```python
from build123d import *

# Parameters (mm, degrees)
CROQUIS1_W              = 34
CROQUIS1_H              = 34
CROQUIS1_R              = 1
SALIENTE_EXTRUIR1_DEPTH = 1
CROQUIS2_W              = 9.310717014
CROQUIS2_H              = 8.671746239
CROQUIS2_W_2            = 1.095378472
CROQUIS2_H_2            = 1.688708478
CROQUIS2_W_3            = 1.004096933
CROQUIS2_H_3            = 1.734349248
SALIENTE_EXTRUIR2_DEPTH = 1


with BuildPart() as part:
    # Croquis1 → Saliente-Extruir1 (new body)
    with BuildSketch(Plane.XY):
        with Locations((17, 17)):
            Rectangle(CROQUIS1_W, CROQUIS1_H)
        with Locations((1.5, 32.5)):
            Circle(CROQUIS1_R, mode=Mode.SUBTRACT)
        with Locations((32.5, 32.5)):
            Circle(CROQUIS1_R, mode=Mode.SUBTRACT)
        with Locations((1.5, 1.5)):
            Circle(CROQUIS1_R, mode=Mode.SUBTRACT)
        with Locations((32.5, 1.5)):
            Circle(CROQUIS1_R, mode=Mode.SUBTRACT)
    extrude(amount=SALIENTE_EXTRUIR1_DEPTH)

    # Croquis2 → Saliente-Extruir2 (add)
    with BuildSketch(Plane.XY.offset(1)):
        with Locations((16.771796152, 16.520771918)):
            Rectangle(CROQUIS2_W, CROQUIS2_H)
        with Locations((14.033349971, 21.700999277)):
            Rectangle(CROQUIS2_W_2, CROQUIS2_H_2)
        with Locations((19.373320023, 21.700999277)):
            Rectangle(CROQUIS2_W_3, CROQUIS2_H_2)
        with Locations((14.033349971, 11.317724175)):
            Rectangle(CROQUIS2_W_2, CROQUIS2_H_3)
        with Locations((19.373320023, 11.317724175)):
            Rectangle(CROQUIS2_W_3, CROQUIS2_H_3)
    extrude(amount=SALIENTE_EXTRUIR2_DEPTH)


solid = part.part
```
The model under review builds one solid part; all positions refer to its coordinate system, in mm. A direction names the side the tool comes from. Round coordinates to 2 decimals unless told otherwise and drop trailing zeros. Write each loop counter-clockwise with the first axis right and the second up, starting at its lowest first coordinate (ties: lowest second). Pieces come first, ordered by that corner, then holes.
(1) Insertion check: pin 1 (0.5 mm diameter, centred on y = 11, z = 1.5, fed in from -X); pin 2 (0.8 mm diameter, centred on x = 19.5, z = 1.5, fed in from -Y); pin 3 (0.8 mm diameter, centred on x = 17.5, z = 1.5, fed in from -Y). Each pin has a flat end and moves straight along its axis. Give the tip position at first contact, or say it passes through.
(2) We need section D-D on y = 22. Give the boundary of the cut face in (x, z), and give its area (3 significant figures).
(3) We need section A-A on y = 1.5. Give the boundary of the cut face in (x, z).
(4) We need section C-C on z = 1.7. Give the boundary of the cut face in (x, y).
(5) Mouldability with a two-part tool opening along Y and no side actions: class faces 4 (the flat face through (18.871, 21.7, 1.5)), 5 (the flat face through (16.7, 20.857, 1.5)), 6 (the cylindrical face through (2.04, 33.34, 0.49)) as +Y half, -Y half, draft (parallel to the pull), parting line (faces both ways), or undercut.
(6) Wall thickness on L1, parallel to Y at x = 32.5, z = 0.45; L2, parallel to Z at x = 7, y = 32.5; L3, parallel to Y at x = 13, z = 1.55: over which ranges is each line inside the solid? List them lowest first.
(7) Machinability: for faces 1 (the flat face through (13.486, 21.7, 1.5)), 2 (the flat face through (12.116, 16.5, 1.5)), 3 (the flat face through (19.4, 22.545, 1.5)), which of the approach directions +Z, -Z, +X, -X, +Y, -Y give a long, thin tool a straight path to every point of the face, cutting with its end or side? Answer none if there is none.
Findings below:
1. pin 1: stops at x = 13.49
1. pin 2: stops at y = 10.45
1. pin 3: stops at y = 12.18
2. outline: (0, 0) - (34, 0) - (34, 1) - (19.88, 1) - (19.88, 2) - (18.87, 2) - (18.87, 1) - (14.58, 1) - (14.58, 2) - (13.49, 2) - (13.49, 1) - (0, 1) - close
2. area: 36.1 mm2
3. outline: (0, 0) - (0.5, 0) - (0.5, 1) - (0, 1) - close; (2.5, 0) - (31.5, 0) - (31.5, 1) - (2.5, 1) - close; (33.5, 0) - (34, 0) - (34, 1) - (33.5, 1) - close
4. outline: (12.12, 12.18) - (13.49, 12.18) - (13.49, 10.45) - (14.58, 10.45) - (14.58, 12.18) - (18.87, 12.18) - (18.87, 10.45) - (19.88, 10.45) - (19.88, 12.18) - (21.43, 12.18) - (21.43, 20.86) - (19.88, 20.86) - (19.88, 22.55) - (18.87, 22.55) - (18.87, 20.86) - (14.58, 20.86) - (14.58, 22.55) - (13.49, 22.55) - (13.49, 20.86) - (12.12, 20.86) - close
5. face 4: draft
5. face 5: +Y half
5. face 6: undercut
6. L1: y = 0 to 0.5, 2.5 to 31.5, 33.5 to 34
6. L2: z = 0 to 1
6. L3: y = 12.18 to 20.86
7. face 1: +Z, -X, +Y
7. face 2: +Z, -X, +Y, -Y
7. face 3: +Z, +X, -X, +Y
